from build123d import *

# Parameters (mm, degrees)
BOSS_EXTRUDE6_DEPTH = 11
SKETCH4_W           = 25
SKETCH4_H           = 11
SKETCH4_H_2         = 11.1
CUT_EXTRUDE1_DEPTH  = 12
FILLET1_R           = 25
FILLET2_R           = 5


with BuildPart() as part:
    # Sketch1 → Boss-Extrude6 (new body)
    with BuildSketch(Plane(origin=(0, 0, 0), x_dir=(1, 0, 0), z_dir=(0, 1, 0))):
        with BuildLine():
            Line((0, -7.5), (125, -7.5))
            Line((125, -7.5), (125, 3.5))
            Line((125, 3.5), (155, 33.5))
            Line((155, 33.5), (155, 123.5))
            Line((155, 123.5), (65.5, 123.5))
            Line((65.5, 123.5), (65.5, 99.705746838))
            ThreePointArc((65.5, 99.705746838), (62.5, 96.705746838), (59.5, 99.705746838))
            Line((59.5, 99.705746838), (59.5, 123.5))
            Line((59.5, 123.5), (-30, 123.5))
            Line((-30, 123.5), (-30, 33.5))
            Line((-30, 33.5), (0, 3.5))
            Line((0, 3.5), (0, -7.5))
        make_face()
        with BuildLine():
            Line((137, 63.5), (137, 93.5))
            ThreePointArc((137, 93.5), (140, 96.5), (143, 93.5))
            Line((143, 93.5), (143, 63.5))
            ThreePointArc((143, 63.5), (140, 60.5), (137, 63.5))
        make_face(mode=Mode.SUBTRACT)
        with BuildLine():
            Line((-18, 63.5), (-18, 93.5))
            ThreePointArc((-18, 93.5), (-15, 96.5), (-12, 93.5))
            Line((-12, 93.5), (-12, 63.5))
            ThreePointArc((-12, 63.5), (-15, 60.5), (-18, 63.5))
        make_face(mode=Mode.SUBTRACT)
        with BuildLine():
            Line((59.5, 16), (59.5, 46))
            ThreePointArc((59.5, 46), (62.5, 49), (65.5, 46))
            Line((65.5, 46), (65.5, 16))
            ThreePointArc((65.5, 16), (62.5, 13), (59.5, 16))
        make_face(mode=Mode.SUBTRACT)
    extrude(amount=BOSS_EXTRUDE6_DEPTH)

    # Sketch4 → Cut-Extrude1 (cut, through all)
    with BuildSketch(Plane(origin=(0, 11, 0), x_dir=(1, 0, 0), z_dir=(0, 1, 0))):
        with Locations((12.5, -2)):
            Rectangle(SKETCH4_W, SKETCH4_H)
        with Locations((62.5, -2)):
            Rectangle(SKETCH4_W, SKETCH4_H)
        with Locations((12.5, 75)):
            Rectangle(SKETCH4_W, SKETCH4_H_2)
        with Locations((112.5, -2)):
            Rectangle(SKETCH4_W, SKETCH4_H)
        with Locations((62.5, 75)):
            Rectangle(SKETCH4_W, SKETCH4_H_2)
        with Locations((112.5, 75)):
            Rectangle(SKETCH4_W, SKETCH4_H_2)
    extrude(amount=-CUT_EXTRUDE1_DEPTH, mode=Mode.SUBTRACT)

    # Fillet1
    fillet1_edges = [part.edges().sort_by_distance(p)[0] for p in [
        (-30, 5.5, -123.5),
        (155, 5.5, -123.5),
    ]]
    fillet(fillet1_edges, radius=FILLET1_R)

    # Fillet2
    fillet2_edges = [part.edges().sort_by_distance(p)[0] for p in [
        (0, 5.5, -3.5),
        (-30, 5.5, -33.5),
        (155, 5.5, -33.5),
        (125, 5.5, -3.5),
    ]]
    fillet(fillet2_edges, radius=FILLET2_R)


solid = part.part
Can you work these out from the model? Positions are in its coordinate system, mm. A direction names the side the tool comes from. Give positions to 0.01 mm unless a question says otherwise; leave off trailing zeros. Order: outer loops, then holes, each group sorted by start corner. A loop starts at its lowest first (then second) coordinate and runs counter-clockwise, first axis right, second up. Notation, with made-up numbers: M -36.75,49.25 L -13.75,49.25 A29 cw -13.75,75.25 Z; hole C 81.5,1.25 d3. An arc over 180 degrees is marked long. One line per question, with ' | ' between items.
Item 1: Suppose I cut it at C-C, the plane x = 117.5. Write out the boundary of the cut face in (y, z).
Answer block:
outline: M 0,-123.5 L 11,-123.5 L 11,-80.55 L 0,-80.55 Z; M 0,-69.45 L 11,-69.45 L 11,-3.5 L 0,-3.5 Z
Item 2: Please list where these lines run through material, in increasing order: L1, parallel to X at y = 6, z = -70; L2, parallel to Z at x = 107.5, y = 2; L3, parallel to X at y = 5, z = -35.
Answer block:
L1: x = -30 to -18, -12 to 0, 25 to 50, 75 to 100, 125 to 137, 143 to 155 | L2: z = -123.5 to -80.55, -69.45 to -3.5 | L3: x = -29.97 to 59.5, 65.5 to 154.97
Item 3: I'm going to push flat-ended pins straight in: pin 1 Ø1 at (x, y) = (105.5, 8) entering from +Z; pin 2 Ø5.5 at (y, z) = (8, -0.5) entering from +X. Where does each tip first touch, or does it pass through?
Answer block:
pin 1: stops at z = -3.5 | pin 2: stops at x = 100
Item 4: We'd pull the mould along Z, two halves only. Please class faces 5 (the face through (65.5, 5, -112)), 6 (the face through (112, 6, -69.45)), 7 (the face through (112, 6, -80.55)), 8 (the face through (28, 5, -123.5)): released by +Z, released by -Z, zero draft, split by the parting line, or undercut.
Answer block:
face 5: zero draft | face 6: undercut | face 7: undercut | face 8: released by -Z
Item 5: Suppose I cut it at D-D, the plane z = -26. Write out the boundary of the cut face in (x, y), then the cut area to 3 significant figures.
Answer block:
outline: M -22.5,0 L 59.5,0 L 59.5,11 L -22.5,11 Z; M 65.5,0 L 147.5,0 L 147.5,11 L 65.5,11 Z | area: 1,800 mm2
Item 6: Suppose I cut it at A-A, the plane z = -67. Write out the boundary of the cut face in (x, y).
Answer block:
outline: M -30,0 L -18,0 L -18,11 L -30,11 Z; M -12,0 L 137,0 L 137,11 L -12,11 Z; M 143,0 L 155,0 L 155,11 L 143,11 Z
Item 7: For faces 1 (the face through (59.5, 5, -111)), 2 (the face through (50, 6, -75)), 3 (the face through (50, 6, 2)), 4 (the face through (61, 11, -59)), which set-ups out of +Z, -Z, +X, -X, +Y, -Y let a thin tool reach every point of the face, with its end or its side?
Answer block:
face 1: -Z, +Y, -Y | face 2: +Y, -Y | face 3: +Z, +Y, -Y | face 4: +Z, -Z, +X, -X, +Y
Item 8: Suppose I cut it at B-B, the plane x = 62.5. Write out the boundary of the cut face in (y, z), then the cut area to 3 significant figures.
Answer block:
outline: M 0,-96.71 L 11,-96.71 L 11,-80.55 L 0,-80.55 Z; M 0,-69.45 L 11,-69.45 L 11,-49 L 0,-49 Z; M 0,-13 L 11,-13 L 11,-3.5 L 0,-3.5 Z | area: 507 mm2
